For this review, take the finished solid that the model builds, in its own axes (mm). A direction names the side the tool comes from. Give positions to 0.01 mm unless a question says otherwise; leave off trailing zeros. Loops run counter-clockwise (first coordinate to the right, second up) from the corner with the lowest first, then second, coordinate; pieces in that order, holes last. Notation, with made-up numbers: (58.5, 64.25) -> (66.5, 64.25) arc R24 ccw to (66.5, 96.25) -> close; hole circle Ø10 at (-28.75, 45.25). An arc over 180 degrees is marked (long way). One line per question, with ' | ' between items. Start each with the question number.
(1) Wall thickness on probe 1 along Z at (x, y) = (-6, -26.05); probe 2 along Y at (x, z) = (-6.25, 14); probe 3 along Y at (x, z) = (-13.75, 7): over which ranges is each line inside the solid? List them lowest first.
(2) Draft analysis for pull direction Z (two halves, no side actions). For faces 6 (the cylindrical face through (-8.1, 23.17, 14.27)), 7 (the flat face through (-8, 18.35, 10)), 8 (the cylindrical face through (-7.895, 0.899, -8.146)), state which applies: +Z half, -Z half, draft (parallel to the pull), parting line (faces both ways), or undercut.
(3) Consider section A-A (y = -26.05). Write out the cut boundary in (x, z).
(4) Consider section D-D (z = 8.5). Write out the cut boundary in (x, y).
(5) Consider section B-B (x = -11.5). Give the number of separate pieces and of enclosed holes in the cut face, and give its area (3 significant figures).
(6) Insertion check: P1, Ø1.6, axis at x = -9.5, y = -16, coming from the +Z side; P2, Ø12, axis at y = -12, z = 16.5, coming from the -X side; P3, Ø1.4, axis at x = -6.5, z = -5.5, coming from the +Y side; P4, Ø6, axis at x = -4.5, y = -20, coming from the +Z side. Each pin has a flat end and moves straight along its axis. Give the tip position at first contact, or say it passes through.
(7) Tool access review of faces 1 (the flat face through (-8, -25, 19.5)), 2 (the flat face through (-8, 1.5, -5)), 3 (the flat face through (-8, -22.45, 10)), 4 (the flat face through (-8, -29.45, 9)), 5 (the flat face through (-8, -24, -2)): name each direction out of +Z, -Z, +X, -X, +Y, -Y from which nothing blocks a thin tool from reaching the whole face with its end or side.
(8) Consider section C-C (z = 14). Write out the cut boundary in (x, y).
Autodesk Inventor part; units mm, degrees
ref_plane "XZ Plane" through (0, 0, 0) normal (0, 1, 0) x (-1, 0, 0)
ref_plane "XY Plane" through (0, 0, 0) normal (0, 0, 1) x (1, 0, 0)
ref_plane "Work Plane1" through (-15.5, 0, 0) normal (1, 0, 0) x (0, 1, 0)
sketch "Sketch1" plane through (-15.5, 0, 0) normal (1, 0, 0) x (0, 1, 0)
  line L0 (-0.5, 0) -> (-0.5, -6.716667)
  line L1 (-0.5, -6.716667) -> (-15.5, -6.716667)
  line L2 (-17, -7) -> (-15.5, -7)
  line L3 (-17, 0) -> (-17, -7)
  line L4 (-17, 0) -> (-22.45, 0)
  line L5 (-22.45, 0) -> (-22.45, 19.5)
  line L6 (-22.45, 19.5) -> (-29.45, 19.5)
  line L7 (-29.45, 19.5) -> (-29.45, -2)
  line L8 (-29.45, -2) -> (-19, -2)
  line L9 (-19, -2) -> (-19, -8.716667)
  line L10 (-19, -8.716667) -> (1.5, -8.716667)
  line L11 (-17, -7) -> (-0.5, -7) construction
  line L12 (-9.247706, -7) -> (-9.247706, -16.201099) construction
  line L13 (1.5, -8.716667) -> (1.5, -2)
  line L14 (1.5, -2) -> (25.35, -2)
  line L15 (25.35, -2) -> (25.35, 19.691667)
  line L16 (25.35, 19.691667) -> (18.35, 19.691667)
  line L17 (18.35, 19.691667) -> (18.35, 0)
  line L18 (18.35, 0) -> (0, 0)
  line L19 (-14.45, -1.808333) -> (-14.45, -5.115) construction
  dimension "d1" = 19.5
  dimension "d2" = 2
  dimension "d3" = 2
  dimension "d4" = 2
  dimension "d5" = 7
  dimension "d6" = 7
  dimension "d7" = 2
  dimension "d8" = 8
  dimension "d9" = 40.8
sketch "Sketch1 outline for Extrusion1" plane through (-15.5, 0, 0) normal (1, 0, 0) x (0, 1, 0)
  line L0 (-17, 0) -> (-22.45, 0)
  line L1 (-17, -7) -> (-17, 0)
  line L2 (-15.5, -7) -> (-17, -7)
  line L3 (-0.5, -6.716667) -> (-15.5, -7)
  line L4 (0, 0) -> (-0.5, -6.716667)
  line L5 (18.35, 0) -> (0, 0)
  line L6 (18.35, 19.691667) -> (18.35, 0)
  line L7 (25.35, 19.691667) -> (18.35, 19.691667)
  line L8 (25.35, -2) -> (25.35, 19.691667)
  line L9 (1.5, -2) -> (25.35, -2)
  line L10 (1.5, -8.716667) -> (1.5, -2)
  line L11 (-19, -8.716667) -> (1.5, -8.716667)
  line L12 (-19, -2) -> (-19, -8.716667)
  line L13 (-29.45, -2) -> (-19, -2)
  line L14 (-29.45, 19.5) -> (-29.45, -2)
  line L15 (-22.45, 19.5) -> (-29.45, 19.5)
  line L16 (-22.45, 0) -> (-22.45, 19.5)
extrude "Extrusion1" add sketch "Sketch1 outline for Extrusion1" along normal blind 15
sketch "Sketch2" plane through (-0.5, 0, 0) normal (1, 0, 0) x (0, 0, -1)
  line L0 (0, -17) -> (0, -22.45)
  line L1 (0, 18.35) -> (0, 0)
  line L2 (-19.5, -29.45) -> (2, -29.45)
  line L3 (2, 25.35) -> (-19.691667, 25.35)
  point P0 (-4.5, -26.05)
  point P1 (-14, -26.05)
  point P2 (-4.5, 21.95)
  point P3 (-14, 21.95)
  dimension "d12" = 4.5
  dimension "d13" = 9.5
  dimension "d14" = 4.5
  dimension "d15" = 9.5
  dimension "d16" = 48
  dimension "d17" = 3.4
  dimension "d18" = 3.4
hole "Hole1" at (-0.5, -26.05, 4.5) at (-0.5, -26.05, 14) at (-0.5, 21.95, 4.5) at (-0.5, 21.95, 14) direction (-1, 0, 0) diameter 2.5 end through all
fillet "Fillet1" radius 2 8 edges at (-8, 25.35, 19.6917) (-8, 25.35, -2) (-8, 1.5, -2) (-8, 1.5, -8.7167) (-8, -19, -8.7167) (-8, -29.45, -2) (-8, -29.45, 19.5) (-8, -19, -2)
equation "\"d2\" = d3"
equation "\"d4\" = d3"
equation "\"d7\" = d3"
properties part number "bracket"
A:
1) probe 1: z = -2 to 3.25, 5.75 to 12.75, 15.25 to 19.5 | probe 2: y = -29.45 to -27.3, -24.8 to -22.45, 18.35 to 20.7, 23.2 to 25.35 | probe 3: y = -29.45 to -22.45, 18.35 to 25.35
2) face 6: undercut | face 7: draft | face 8: -Z half
3) outline: (-15.5, -2) -> (-0.5, -2) -> (-0.5, 3.25) -> (-15.5, 3.25) -> close; (-15.5, 5.75) -> (-0.5, 5.75) -> (-0.5, 12.75) -> (-15.5, 12.75) -> close; (-15.5, 15.25) -> (-0.5, 15.25) -> (-0.5, 19.5) -> (-15.5, 19.5) -> close
4) outline: (-15.5, -29.45) -> (-0.5, -29.45) -> (-0.5, -22.45) -> (-15.5, -22.45) -> close; (-15.5, 18.35) -> (-0.5, 18.35) -> (-0.5, 25.35) -> (-15.5, 25.35) -> close
5) separate pieces: 1 | enclosed holes: 4 | area: 384 mm^2
6) P1: stops at z = -6.99 | P2: passes through | P3: stops at y = 1.5 | P4: stops at z = 19.5
7) face 1: +Z, +X, -X, -Y | face 2: -Z, +X, -X, +Y | face 3: +Z, +X, -X | face 4: +Z, -Z, +X, -X, -Y | face 5: -Z, +X, -X, -Y
8) outline: (-15.5, -29.45) -> (-0.5, -29.45) -> (-0.5, -27.3) -> (-15.5, -27.3) -> close; (-15.5, -24.8) -> (-0.5, -24.8) -> (-0.5, -22.45) -> (-15.5, -22.45) -> close; (-15.5, 18.35) -> (-0.5, 18.35) -> (-0.5, 20.7) -> (-15.5, 20.7) -> close; (-15.5, 23.2) -> (-0.5, 23.2) -> (-0.5, 25.35) -> (-15.5, 25.35) -> close
